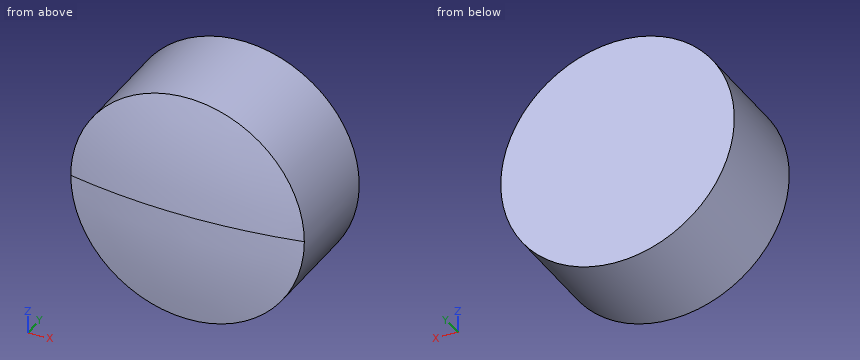
```python
from build123d import *

# Parameters (mm, degrees)
F2_R          = 51.3419561809
F2_R_2        = 6.35
F3_DEPTH      = 31.751
F3_DEPTH_BACK = 31.751
F4_R          = 20.622673328
F5_DEPTH      = 31.751
F5_DEPTH_BACK = 25.4


with BuildPart() as f1:
    # F0 (on Front) → F1 (revolve)
    with BuildSketch(Plane.XZ):
        with BuildLine():
            ThreePointArc((0, -31.75), (22.4506403027, -22.4506403027), (31.75, 0))
            ThreePointArc((31.75, 0), (22.4506403027, 22.4506403027), (0, 31.75))
            Line((0, 31.75), (0, -31.75))
        make_face()
    revolve(axis=Axis((0, 0, 0), (0, 0, -1)))

    # F2 (on Front) → F3 (cut, two sides)
    with BuildSketch(Plane.XZ) as f3_sk:
        Circle(F2_R)
        Circle(F2_R_2, mode=Mode.SUBTRACT)
    extrude(amount=-F3_DEPTH, mode=Mode.SUBTRACT)
    extrude(f3_sk.sketch, amount=F3_DEPTH_BACK, mode=Mode.SUBTRACT)

    # F4 (on Front) → F5 (cut, two sides)
    with BuildSketch(Plane.XZ) as f5_sk:
        Circle(F4_R)
    extrude(amount=-F5_DEPTH, mode=Mode.SUBTRACT)
    extrude(f5_sk.sketch, amount=F5_DEPTH_BACK, mode=Mode.SUBTRACT)


solid = f1.part
```
The listing builds one solid part. Answer for the finished solid, in the listing's coordinates (mm). Give positions to 0.01 mm unless a question says otherwise; leave off trailing zeros. Order: outer loops, then holes, each group sorted by start corner. A loop starts at its lowest first (then second) coordinate and runs counter-clockwise, first axis right, second up.
1) Consider line 1 along X through (y, z) = (-25.75, -2.5); line 2 along X through (y, z) = (-31, 3.25); line 3 along Y through (x, z) = (-4.25, 1.25). Determine where each line is inside the solid, lowest interval first.
Reported:
line 1: x = -5.84 to 5.84
line 2: x = -5.46 to 5.46
line 3: y = -31.44 to -25.4
2) Find section B-B on y = -27. Write down the section's boundary in (x, z).
Reported:
outline: circle Ø12.7 at (0, 0)
3) Find section D-D on x = -4.5. Write down the section's boundary in (y, z), then the cut area to 3 significant figures.
Reported:
outline: (-31.11, -4.48) - (-25.4, -4.48) - (-25.4, 4.48) - (-31.11, 4.48) arc R31.43 ccw to start
area: 53.1 mm2
4) Given P1, Ø3, axis at y = -29, z = 3, coming from the -X side; P2, Ø1, axis at x = -4, y = -30.5, coming from the +Z side; P3, Ø3, axis at x = -4, y = -29.5, coming from the -Z side, each flat-ended and moving along its own axis, determine where each tip first touches the part or whether it passes through.
Reported:
P1: stops at x = -6.17
P2: stops at z = 5.3
P3: stops at z = -5.84
5) Find section A-A on x = 0. Write down the section's boundary in (y, z).
Reported:
outline: (-31.11, -6.35) - (-25.4, -6.35) - (-25.4, 6.35) - (-31.11, 6.35) arc R31.75 ccw to start
6) Find section C-C on z = -0.5. Write down the section's boundary in (x, y), then the cut area to 3 significant figures.
Reported:
outline: (-6.33, -31.11) arc R31.75 ccw to (6.33, -31.11) - (6.33, -25.4) - (-6.33, -25.4) - close
area: 77.7 mm2
